Design review of the part built by this model. Coordinates are the model's own, in mm. Coordinates: 2 decimals unless noted, no trailing zeros. Write each loop counter-clockwise with the first axis right and the second up, starting at its lowest first coordinate (ties: lowest second). Pieces come first, ordered by that corner, then holes. Notation, with made-up numbers: M 83,-14 L 104,-14 A18 ccw 104,-1 Z; hole C 87,59.25 d6. An arc over 180 degrees is marked long. One line per question, with ' | ' between items.
from build123d import *

# Parameters (mm, degrees)
F0_R     = 63.5
F1_DEPTH = 3.429
F2_SIZE  = 19.05


with BuildPart() as f1:
    # F0 (on Front) → F1 (new body)
    with BuildSketch(Plane.XZ):
        Polygon((103.9749, -16.129), (103.9749, 110.871), (-103.9749, 110.871), (-103.9749, -110.871), (107.2769, -110.871), (107.2769, -16.129), align=None)
        Circle(F0_R, mode=Mode.SUBTRACT)
    extrude(amount=F1_DEPTH)

    # F2
    f2_edges = [f1.edges().sort_by_distance(p)[0] for p in [
        (-103.9749, -1.7145, 110.871),
        (103.9749, -1.7145, 110.871),
        (107.2769, -1.7145, -110.871),
        (-103.9749, -1.7145, -110.871),
    ]]
    chamfer(f2_edges, length=F2_SIZE)


solid = f1.part
1. Take a section at A-A (z = 0). Write out the cut boundary in (x, y).
Answer sheet:
outline: M -103.97,-3.43 L -63.5,-3.43 L -63.5,0 L -103.97,0 Z; M 63.5,-3.43 L 103.97,-3.43 L 103.97,0 L 63.5,0 Z
2. To check wall thickness, follow line 1 along Z through (x, y) = (0, -1.4); line 2 along Z through (x, y) = (49, -3.15); line 3 along X through (y, z) = (-2.9, 83). State the ranges of each line that lie inside material, in increasing order. Write a range as [from, to].
Answer sheet:
line 1: [-110.87, -63.5], [63.5, 110.87] | line 2: [-110.87, -40.39], [40.39, 110.87] | line 3: [-103.97, 103.97]
3. Take a section at C-C (y = -1.45). Write out the cut boundary in (x, z).
Answer sheet:
outline: M -103.97,-91.82 L -84.92,-110.87 L 88.23,-110.87 L 107.28,-91.82 L 107.28,-16.13 L 103.97,-16.13 L 103.97,91.82 L 84.92,110.87 L -84.92,110.87 L -103.97,91.82 Z; hole C 0,0 d127
4. Insertion check: pin 1 Ø1.7 at (x, y) = (105, -1.5) entering from +Z; pin 2 Ø1.7 at (y, z) = (-2, 46.5) entering from +X. Each pin has a flat end and moves straight along its axis. Give the tip position at first contact, or say it passes through.
Answer sheet:
pin 1: z = -16.13 | pin 2: x = 103.97
5. Take a section at B-B (x = 0). Write out the cut boundary in (y, z).
Answer sheet:
outline: M -3.43,-110.87 L 0,-110.87 L 0,-63.5 L -3.43,-63.5 Z; M -3.43,63.5 L 0,63.5 L 0,110.87 L -3.43,110.87 Z
6. Draft analysis for pull direction Z (two halves, no side actions). For faces 1 (the face through (-13.77, -1.69, -61.99)), 2 (the face through (-47, -3.429, 51)), 3 (the face through (-94.583, -1.69, 101.213)), state which applies: pulls with the +Z half, pulls with the -Z half, needs draft (parallel to the pull), parting line crosses it, or undercut.
Answer sheet:
face 1: undercut | face 2: needs draft | face 3: pulls with the +Z half
7. Take a section at D-D (z = 83). Write out the cut boundary in (x, y).
Answer sheet:
outline: M -103.97,-3.43 L 103.97,-3.43 L 103.97,0 L -103.97,0 Z
